from build123d import *

# Parameters (mm, degrees)
F1_DEPTH = 3.81
F2_R     = 3.175
F3_DEPTH = 50.8


with BuildPart() as f1:
    # F0 (on Right) → F1 (new body)
    with BuildSketch(Plane.YZ):
        Polygon((-3.666174, -6.35), (3.666174, -6.35), (7.332348, 0), (3.666174, 6.35), (-3.666174, 6.35), (-7.332348, 0), align=None)
    extrude(amount=F1_DEPTH)

    # F2 (on Right) → F3 (join)
    with BuildSketch(Plane.YZ):
        Circle(F2_R)
    extrude(amount=-F3_DEPTH)


solid = f1.part
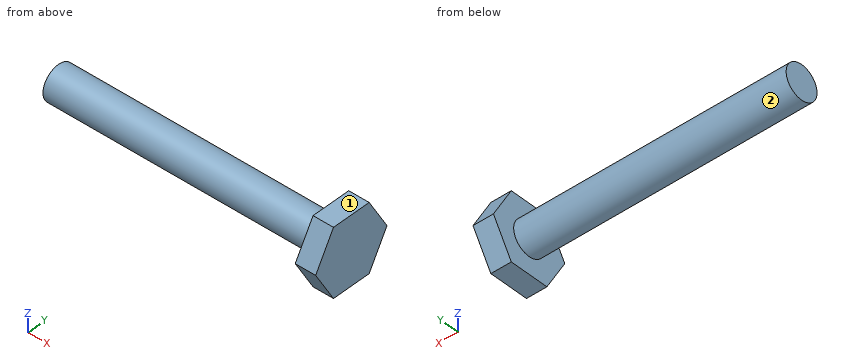
Can you work these out from the model? Positions are in its coordinate system, mm. Face numbers are marked on the shaded views. A direction names the side the tool comes from. Round coordinates to 2 decimals unless told otherwise and drop trailing zeros. Write each loop counter-clockwise with the first axis right and the second up, starting at its lowest first coordinate (ties: lowest second). Pieces come first, ordered by that corner, then holes. Notation, with made-up numbers: (13, -7) -> (53, -7) arc R9 cw to (53, 8) -> close; hole circle Ø4 at (68, 71). An arc over 180 degrees is marked (long way). Use one line per item in the form item = value. Start each with the question number.
Q1. If I drill on probe 1 along X at (y, z) = (3, -3.75); probe 2 along Y at (x, z) = (-31.5, -0.25); probe 3 along Z at (x, y) = (-9, 1.25), over which ranges is the centre line in solid material (lowest first)? Write a range as [from, to].
Q2. I'm going to push flat-ended pins straight in: P1, Ø1.5, axis at x = -24, z = -1, coming from the +Y side; P2, Ø5, axis at x = -20, z = -5, coming from the +Y side; P3, Ø1.5, axis at x = -19, z = -2.5, coming from the -Y side. Where does each tip first touch, or does it pass through?
Q3. Imagine slicing it at C-C (x = -38.5). Please give me the cut outline in (y, z) (3 decimals), then the cut area to 3 significant figures.
Q4. Which directions (+Z, -Z, +X, -X, +Y, -Y) give clear straight access to the entire face, cutting with the end or side of a thin tool? Please do the marked faces 1 and 2.
Q5. Imagine slicing it at D-D (y = 4.75). Please give me the cut outline in (x, z).
Q6. Imagine slicing it at B-B (z = -2.5). Please give me the cut outline in (x, y).
Q7. Imagine slicing it at A-A (y = 0). Please give me the cut outline in (x, z) (3 decimals).
Worked out:
q1.probe_1 = [0, 3.81]
q1.probe_2 = [-3.17, 3.17]
q1.probe_3 = [-2.92, 2.92]
q2.P1 = 3.17
q2.P2 = 1.96
q2.P3 = -2.65
q3.outline = circle Ø6.35 at (0, 0)
q3.area = 31.7 mm^2
q4.face_1 = +Z, +X, -X, +Y, -Y
q4.face_2 = -X
q5.outline = (0, -4.47) -> (3.81, -4.47) -> (3.81, 4.47) -> (0, 4.47) -> close
q6.outline = (-50.8, -1.96) -> (0, -1.96) -> (0, -5.89) -> (3.81, -5.89) -> (3.81, 5.89) -> (0, 5.89) -> (0, 1.96) -> (-50.8, 1.96) -> close
q7.outline = (-50.8, -3.175) -> (0, -3.175) -> (0, -6.35) -> (3.81, -6.35) -> (3.81, 6.35) -> (0, 6.35) -> (0, 3.175) -> (-50.8, 3.175) -> close
